```python
from build123d import *

# Parameters (mm, degrees)
SKETCH1_W           = 25.4
SKETCH1_H           = 12.7
BOSS_EXTRUDE1_DEPTH = 76.2
FILLET1_R           = 6.35
SKETCH3_W           = 18.288
SKETCH3_H           = 6.858
SKETCH3_W_2         = 17.78
SKETCH3_H_2         = 6.35
BOSS_EXTRUDE2_DEPTH = 17.78
SKETCH4_W           = 17.78
SKETCH4_H           = 3.175
BOSS_EXTRUDE3_DEPTH = 17.526
SKETCH5_W           = 2.54
SKETCH5_H           = 2.54
CUT_EXTRUDE1_DEPTH  = 0.254
SKETCH7_W           = 2.54
SKETCH7_H           = 2.54
CUT_EXTRUDE6_DEPTH  = 0.254
FILLET2_R           = 0.762
FILLET3_R           = 0.762
SKETCH20_R          = 7.62
BOSS_EXTRUDE4_DEPTH = 1.27
BOSS_EXTRUDE5_START = 1.27
SKETCH21_R          = 7.62
BOSS_EXTRUDE5_DEPTH = 1.27
SKETCH23_W          = 3.136693438
SKETCH23_H          = 1.456321954
BOSS_EXTRUDE6_DEPTH = 0.254


with BuildPart() as part:
    # Sketch1 → Boss-Extrude1 (new body)
    with BuildSketch(Plane.XY):
        Rectangle(SKETCH1_W, SKETCH1_H)
    extrude(amount=BOSS_EXTRUDE1_DEPTH)

    # Fillet1
    fillet1_edges = [part.edges().sort_by_distance(p)[0] for p in [
        (0, 6.35, 0),
        (0, -6.35, 0),
    ]]
    fillet(fillet1_edges, radius=FILLET1_R - 0.0001)  # a hair under: the kernel refuses the full size

    # Sketch3 → Boss-Extrude2 (add)
    with BuildSketch(Plane.XY.offset(76.2)):
        Rectangle(SKETCH3_W, SKETCH3_H)
        Rectangle(SKETCH3_W_2, SKETCH3_H_2, mode=Mode.SUBTRACT)
    extrude(amount=BOSS_EXTRUDE2_DEPTH)

    # Sketch4 → Boss-Extrude3 (add)
    with BuildSketch(Plane.XY.offset(76.2)):
        with Locations((0, -1.5875)):
            Rectangle(SKETCH4_W, SKETCH4_H)
    extrude(amount=BOSS_EXTRUDE3_DEPTH)

    # Sketch5 → Cut-Extrude1 (cut)
    with BuildSketch(Plane(origin=(0, 3.429, 0), x_dir=(1, 0, 0), z_dir=(0, 1, 0))):
        with Locations((4.832637326, -85.369889154)):
            Rectangle(SKETCH5_W, SKETCH5_H)
        with Locations((-4.311362674, -85.369889154)):
            Rectangle(SKETCH5_W, SKETCH5_H)
    extrude(amount=-CUT_EXTRUDE1_DEPTH, mode=Mode.SUBTRACT)

    # Sketch7 → Cut-Extrude6 (cut)
    with BuildSketch(Plane.XZ.offset(3.429)):
        with Locations((4.832637326, 85.369889154)):
            Rectangle(SKETCH7_W, SKETCH7_H)
        with Locations((-4.311362674, 85.369889154)):
            Rectangle(SKETCH7_W, SKETCH7_H)
    extrude(amount=-CUT_EXTRUDE6_DEPTH, mode=Mode.SUBTRACT)

    # Fillet2
    fillet2_edges = [part.edges().sort_by_distance(p)[0] for p in [
        (-12.7, -4.49015735, 1.85984265),
        (-12.7, 4.49015735, 1.85984265),
        (12.7, -4.49015735, 1.85984265),
        (12.7, 4.49015735, 1.85984265),
        (12.7, -6.35, 41.27495),
        (-12.7, -6.35, 41.27495),
        (-12.7, 6.35, 41.27495),
        (12.7, 6.35, 41.27495),
    ]]
    fillet(fillet2_edges, radius=FILLET2_R)

    # Fillet3
    fillet3_edges = [part.edges().sort_by_distance(p)[0] for p in [
        (0, -6.35, 76.2),
        (-12.7, 0, 76.2),
        (12.7, 0, 76.2),
        (0, 6.35, 76.2),
        (12.476815367, 6.126815367, 76.2),
        (-12.476815367, 6.126815367, 76.2),
        (12.476815367, -6.126815367, 76.2),
        (-12.476815367, -6.126815367, 76.2),
    ]]
    fillet(fillet3_edges, radius=FILLET3_R)

    # Sketch20 → Boss-Extrude4 (add)
    with BuildSketch(Plane(origin=(0, 6.35, 0), x_dir=(1, 0, 0), z_dir=(0, 1, 0))):
        with Locations(Location((0, -49.676760647, 0), (0, 0, 90))):
            Circle(SKETCH20_R)
    extrude(amount=BOSS_EXTRUDE4_DEPTH)

    # Sketch21 → Boss-Extrude5 (add)
    with BuildSketch(Plane.XZ.offset(6.35).offset(BOSS_EXTRUDE5_START)):
        with Locations(Location((0, 49.676760647, 0), (0, 0, 270))):
            Circle(SKETCH21_R)
    extrude(amount=-BOSS_EXTRUDE5_DEPTH)

    # Sketch23 → Boss-Extrude6 (add)
    with BuildSketch(Plane(origin=(12.7, 0, 0), x_dir=(0, 0, -1), z_dir=(1, 0, 0))):
        with Locations((-8.954865749, 0)):
            Rectangle(SKETCH23_W, SKETCH23_H)
    extrude(amount=BOSS_EXTRUDE6_DEPTH)


solid = part.part
```
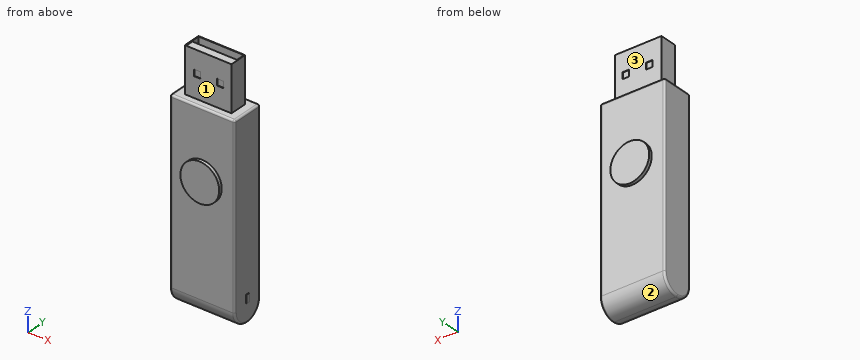
Source: CAD feature listing. Evaluate the final solid. Frame: model axes, mm. Face numbers are marked on the shaded views. A direction names the side the tool comes from. Give positions to 0.01 mm unless a question says otherwise; leave off trailing zeros. Loops run counter-clockwise (first coordinate to the right, second up) from the corner with the lowest first, then second, coordinate; pieces in that order, holes last. Notation, with made-up numbers: (13, 9.25) -> (63, 9.25) arc R32 ccw to (63, 43.25) -> close; hole circle Ø6 at (51.25, 78.5). An arc over 180 degrees is marked (long way). Use a Markdown table: item, result. Add a question column.
(1) Section query C-C (z = 67). Output: boundary loops of the cut face in (x, y), then the cut area to 3 significant figures.
(2) Access query for the marked faces 1, 2 and 3. Directions: +Z, -Z, +X, -X, +Y, -Y. A direction counts if a zero-diameter tool reaches every point of the face in a straight line with its end or side. Return the directions, or none.
(3) First-contact query: pin 1 Ø3 at (y, z) = (1.5, 84.5) entering from -X; pin 2 Ø4 at (x, z) = (8.5, 18) entering from -Y; pin 3 Ø9 at (x, z) = (-4, 87.5) entering from +Y. Flat tips, straight axial feed; report the tip coordinate or a pass-through.
(4) Section query A-A (z = 81). Output: boundary loops of the cut face in (x, y) (3 decimals), then the cut area to 3 significant figures.
(5) Ray query, line 1 (X direction, y = 0.25, z = 35); line 2 (Y direction, x = -0.25, z = 7.5); line 3 (X direction, y = 1.75, z = 80). Return the intervals inside material, ascending.
Checked values:
| question | item | result |
|---|---|---|
| 1 | outline | (-12.7, -5.59) arc R0.76 ccw to (-11.94, -6.35) -> (11.94, -6.35) arc R0.76 ccw to (12.7, -5.59) -> (12.7, 5.59) arc R0.76 ccw to (11.94, 6.35) -> (-11.94, 6.35) arc R0.76 ccw to (-12.7, 5.59) -> close |
| 1 | area | 322 mm^2 |
| 2 | face 1 | +Z, +X, -X, -Y |
| 2 | face 2 | -Z, +X, -X, +Y |
| 2 | face 3 | +Z, +X, -X, +Y |
| 3 | pin 1 | x = -9.14 |
| 3 | pin 2 | y = -6.35 |
| 3 | pin 3 | y = 3.43 |
| 4 | outline | (-9.144, -3.429) -> (9.144, -3.429) -> (9.144, 3.429) -> (-9.144, 3.429) -> close; hole (-8.89, 0) -> (8.89, 0) -> (8.89, 3.175) -> (-8.89, 3.175) -> close |
| 4 | area | 69.0 mm^2 |
| 5 | line 1 | -12.7 to 12.7 |
| 5 | line 2 | -6.35 to 6.35 |
| 5 | line 3 | -9.14 to -8.89, 8.89 to 9.14 |
